```python
from build123d import *

# Parameters (mm, degrees)
REVOLVE_1_ANGLE = 180
SKETCH_6_W      = 9
SKETCH_6_H      = 5
SKETCH_7_W      = 8
SKETCH_7_H      = 4.896318498


with BuildPart() as part:
    # 草图1 → 旋转1 (revolve)
    with BuildSketch(Plane(origin=(0, 0, 0), x_dir=(1, 0, 0), z_dir=(0, 1, 0))):
        with BuildLine():
            Line((0, 9), (0, -9))
            ThreePointArc((0, -9), (9, 0), (0, 9))
        make_face()
    revolve(axis=Axis((0, 0, -9), (0, 0, 1)), revolution_arc=REVOLVE_1_ANGLE)

    # 草图6 → 旋转2 (revolve)
    with BuildSketch(Plane(origin=(0, 0, 0), x_dir=(0, 0, -1), z_dir=(1, 0, 0)), mode=Mode.PRIVATE) as revolve_2_sk:
        with Locations((4.5, -2.5)):
            Rectangle(SKETCH_6_W, SKETCH_6_H)
    revolve(revolve_2_sk.sketch.rotate(Axis((0, 0, 0), (0, -1, 0)), 180), axis=Axis((0, 0, 0), (0, -1, 0)))

    # 草图7 → 切除-旋转2 (revolve, cut)
    with BuildSketch(Plane(origin=(0, 0, 0), x_dir=(0, 0, -1), z_dir=(1, 0, 0)), mode=Mode.PRIVATE) as cut_revolve_2_sk:
        with Locations((4, -2.551840751)):
            Rectangle(SKETCH_7_W, SKETCH_7_H)
    revolve(cut_revolve_2_sk.sketch.rotate(Axis((0, -0.103681502, 0), (0, -1, 0)), 180), axis=Axis((0, -0.103681502, 0), (0, -1, 0)), mode=Mode.SUBTRACT)


solid = part.part
```
Geometry: final body of the model. Coordinates: model frame, mm. Round coordinates to 2 decimals unless told otherwise and drop trailing zeros. Write each loop counter-clockwise with the first axis right and the second up, starting at its lowest first coordinate (ties: lowest second). Pieces come first, ordered by that corner, then holes. Notation, with made-up numbers: M -1,15.5 L 37,15.5 A11 ccw 37,31.5 Z; hole C 3.25,-35 d1. An arc over 180 degrees is marked long. Answer in a Markdown table with one row per item. Add a question column.
(1) Ray query, L1, parallel to X at y = -1.8, z = 0; L2, parallel to Z at x = -1.5, y = -2.25; L3, parallel to Z at x = 2, y = -3.5. Return the intervals inside material, ascending.
(2) Cut plane C-C, the plane y = -1.25. Return the cut outline in (x, z).
(3) Cut plane A-A, the plane x = 0. Return the cut outline in (y, z).
(4) Contact query for flat-ended pins moving along their axis: pin 1 (2 mm diameter, centred on x = -0.5, y = 7, fed in from -Z); pin 2 (8 mm diameter, centred on x = 5.5, z = -0.5, fed in from +Y); pin 3 (6 mm diameter, centred on y = 2.5, z = 2.5, fed in from -X). Output: stop coordinate, or through.
(5) Cut plane B-B, the plane z = 0. Return the cut outline in (x, y), then the cut area to 3 significant figures.
(6) Cut plane D-D, the plane y = 3.5. Return the cut outline in (x, z), then the cut area to 3 significant figures.
(7) Draft query along Z for faces 1 (the face through (0, -0.104, 0)), 2 (the face through (-6.083, -2.465, -6.633)). Return one class per face: pulls with the +Z half, pulls with the -Z half, needs draft (parallel to the pull), parting line crosses it, or undercut.
Established:
| question | item | result |
|---|---|---|
| 1 | L1 | -9 to -8, 8 to 9 |
| 1 | L2 | -8.87 to -7.86, 7.86 to 8.87 |
| 1 | L3 | -8.77 to -7.75, 7.75 to 8.77 |
| 2 | outline | C 0,0 d18; hole C 0,0 d16 |
| 3 | outline | M -5,-9 L 0,-9 A9 ccw 0,9 L -5,9 L -5,8 L -0.1,8 L -0.1,-8 L -5,-8 Z |
| 4 | pin 1 | z = -6.69 |
| 4 | pin 2 | y = 8.87 |
| 4 | pin 3 | x = -8.98 |
| 5 | outline | M -9,-5 L -8,-5 L -8,-0.1 L 8,-0.1 L 8,-5 L 9,-5 L 9,0 A9 ccw -9,0 Z |
| 5 | area | 139 mm² |
| 6 | outline | C 0,0 d16.58 |
| 6 | area | 216 mm² |
| 7 | face 1 | undercut |
| 7 | face 2 | parting line crosses it |
